Build history of the part. All positions in model axes, mm. A direction names the side the tool comes from. Round coordinates to 2 decimals unless told otherwise and drop trailing zeros. Write each loop counter-clockwise with the first axis right and the second up, starting at its lowest first coordinate (ties: lowest second). Pieces come first, ordered by that corner, then holes.
Item 1: Drop flat-ended pins along their axis: pin 1 Ø5.5 at (x, y) = (91, 2) entering from +Z; pin 2 Ø2.5 at (x, y) = (76, 6.5) entering from +Z; pin 3 Ø1.5 at (y, z) = (7.5, -17.5) entering from +X. Give the stop position or say it passes through.
Item 2: Band-saw the part on C-C, the plane x = -82. Write the cut outline in (y, z), then the cut area to 3 significant figures.
Item 3: Band-saw the part on B-B, the plane z = 73.5. Write the cut outline in (x, y), then the cut area to 4 significant figures.
Item 4: Wall check: probe 1 along Z at (x, y) = (82.6, 5.25); probe 2 along Y at (x, z) = (-52, 74.5); probe 3 along Z at (x, y) = (-14, 3.5). Give the ranges that are in metal, low to high.
Item 5: Mould opens along X. For faces 1 (the flat face through (71, 2, 70)), 2 (the flat face through (75, 7, 10.16)), 3 (the flat face through (11.425, 4.507, -23.224)) say: +X half, -X half, draft (parallel to the pull), parting line (faces both ways), or undercut.
Item 6: Band-saw the part on A-A, the plane x = 60. Write the cut outline in (y, z), then the cut area to 3 significant figures.
Item 7: Band-saw the part on D-D, the plane x = -29.5. Write the cut outline in (y, z), then the cut area to 3 significant figures.
Item 8: 3-axis set-ups, long thin cutter, end or side, ignore diameter. For faces 4 (the flat face through (-23.22, 4.51, -22.74)), 5 (the flat face through (75, 7, -23.851)), 6 (the flat face through (10.379, 2.028, -20.027)), 7 (the flat face through (75, 10, -7)), 8 (the flat face through (92, 3, 25.4)): which of +Z, -Z, +X, -X, +Y, -Y reach the whole face in a straight line?
Autodesk Inventor part; units mm, degrees
ref_plane "YZ Plane" through (0, 0, 0) normal (1, 0, 0) x (0, 1, 0)
ref_plane "XZ Plane" through (0, 0, 0) normal (0, 1, 0) x (-1, 0, 0)
ref_plane "XY Plane" through (0, 0, 0) normal (0, 0, 1) x (1, 0, 0)
sketch "Sketch1" plane through (0, 0, 0) normal (0, 1, 0) x (-1, 0, 0)
  line L0 (101.6, -101.6) -> (-101.6, -101.6)
  line L1 (-101.6, -101.6) -> (-101.6, 101.6)
  line L2 (-101.6, 101.6) -> (101.6, 101.6)
  line L3 (101.6, 101.6) -> (101.6, -101.6)
  line L4 (96.6, -96.6) -> (-96.6, -96.6)
  line L5 (-96.6, -96.6) -> (-96.6, 96.6)
  line L6 (-96.6, 96.6) -> (96.6, 96.6)
  line L7 (96.6, 96.6) -> (96.6, -96.6)
  line L8 (101.6, 101.6) -> (-40.4, 101.6)
  circle A0 centre (0, 0) radius 88.9
  line L9 (-40.4, 101.6) -> (-101.6, 40.4)
  line L10 (-45.4, 101.6) -> (-101.6, 45.4)
  line L11 (96.6, 96.6) -> (96.6, 101.6)
  line L12 (-45.4, 101.6) -> (-35.4, 101.6)
  line L13 (-35.4, 101.6) -> (-35.4, 96.6)
  line L14 (-35.4, 96.6) -> (-45.4, 96.6)
  line L15 (-45.4, 96.6) -> (-45.4, 101.6)
  line L16 (-101.6, 39.4) -> (-39.4, 101.6)
  line L17 (95.6, -95.6) -> (-95.6, -95.6)
  line L18 (-95.6, -95.6) -> (-95.6, 95.6)
  line L19 (-95.6, 95.6) -> (95.6, 95.6)
  line L20 (95.6, 95.6) -> (95.6, -95.6)
  point P0 (96.6, 51.2168)
  point P1 (101.6, 40.4)
  point P2 (101.6, -40.4)
  point P3 (96.6, -51.2168)
  point P4 (-96.6, 45.4)
  point P5 (-45.4, 96.6)
  point P6 (-45.4, 95.6)
  point P7 (-95.6, 45.4)
  dimension "d0" = 203.2
  dimension "d1" = 203.2
  dimension "d2" = 101.6
  dimension "d3" = 101.6
  dimension "d4" = 5
  dimension "d5" = 5
  dimension "d6" = 5
  dimension "d7" = 5
  dimension "d8" = 142
  dimension "d9" = 61.2
  dimension "d10" = 177.8
  dimension "d11" = 5
  dimension "d12" = 5
  dimension "d13" = 10
  dimension "d14" = 1
  dimension "d15" = 1
  dimension "d16" = 1
  dimension "d17" = 1
  dimension "d18" = 1
extrude "Extrusion1" add sketch "Sketch1" along normal blind 5 contours L16 L19 L20 L17 L18 | A0
sketch "Sketch2" plane through (0, 5, 0) normal (0, 1, 0) x (1, 0, 0)
  circle A0 centre (0, 0) radius 34.925
  circle A1 centre (0, 0) radius 88.9
  line L0 (0, 0) -> (53.5014, -70.9987)
  line L1 (0, 0) -> (70.9987, -53.5014)
  line L2 (45.4, -95.6) -> (95.6, -45.4)
  line L3 (70.5, -70.5) -> (0, 0)
  point P0 (21.0184, -27.8923)
  point P1 (27.8923, -21.0184)
  dimension "d21" = 69.85
  dimension "d22" = 177.8
  dimension "d23" = 8
  dimension "d24" = 8
extrude "Extrusion2" cut sketch "Sketch2" against normal blind 5 contours A0 L3 A1 L0 | L1 A1 L3 A0
sketch "Sketch3" plane through (0, 5, 0) normal (0, 1, 0) x (1, 0, 0)
  circle A0 centre (0, 0) radius 2.5
  line L0 (11.3314, 2.139) -> (-2.139, -11.3314)
  line L1 (0, 0) -> (-5.6569, 5.6569)
  line L2 (-5.6569, -14.8492) -> (-26.163, 5.6569)
  line L3 (-5.6569, 26.163) -> (14.8492, 5.6569)
  circle A1 centre (-5.6569, 5.6569) radius 14
  line L4 (-26.163, 5.6569) -> (-5.6569, 26.163)
  line L5 (14.8492, 5.6569) -> (-5.6569, -14.8492)
  line L6 (-40.3051, 5.6569) -> (-5.6569, 40.3051)
  line L7 (-5.6569, 40.3051) -> (28.9914, 5.6569)
  line L8 (28.9914, 5.6569) -> (-5.6569, -28.9914)
  line L9 (-5.6569, -28.9914) -> (-40.3051, 5.6569)
  line L10 (-22.6451, 9.1747) -> (-9.1747, 22.6451)
  line L11 (-9.1747, 22.6451) -> (-12.7668, 26.2372)
  line L12 (-12.7668, 26.2372) -> (-26.2372, 12.7668)
  line L13 (-26.2372, 12.7668) -> (-22.6451, 9.1747)
  line L14 (-36.0624, 5.6569) -> (-5.6569, 36.0624)
  line L15 (-5.6569, 36.0624) -> (26.8701, 3.5355)
  line L16 (26.8701, 3.5355) -> (-3.5355, -26.8701)
  line L17 (-3.5355, -26.8701) -> (-36.0624, 5.6569)
  arc A2 (-5.6569, -28.9914) -> (28.9914, 5.6569) centre (0.4206, -0.4206) ccw
  dimension "d27" = 8
  dimension "d28" = 28
  dimension "d29" = 29
  dimension "d30" = 29
  dimension "d31" = 14.5
  dimension "d32" = 10
  dimension "d33" = 10
  dimension "d34" = 10
  dimension "d35" = 10
  dimension "d36" = 5.08
  dimension "d37" = 9.525
  dimension "d38" = 9.525
  dimension "d39" = 3
  dimension "d40" = 3
  dimension "d41" = 0
  dimension "d42" = 3
  dimension "d51" = 29.21
extrude "Extrusion3" cut sketch "Sketch3" against normal blind 1 contours A0 | L0 L5 L2 L4 L3 | L4 L13 L12 L11 | A1 | L6 L7 L8 L15 L14 L17 L9 | L8 A2 | L17 L14 L15 L8
sketch "Sketch4" plane through (0, 4, 0) normal (0, 1, 0) x (1, 0, 0)
  line L0 (-36.0624, 5.6569) -> (-5.6569, 36.0624)
  line L1 (-5.6569, 36.0624) -> (26.8701, 3.5355)
  line L2 (26.8701, 3.5355) -> (-3.5355, -26.8701)
  line L3 (-3.5355, -26.8701) -> (-36.0624, 5.6569)
  line L4 (-5.6569, 40.3051) -> (28.9914, 5.6569)
  line L5 (-40.3051, 5.6569) -> (-5.6569, 40.3051)
  line L6 (-5.6569, -28.9914) -> (-40.3051, 5.6569)
  line L7 (28.9914, 5.6569) -> (-5.6569, -28.9914)
  arc A0 (-3.5355, -26.8701) -> (26.8701, 3.5355) centre (4.0877, -4.0877) ccw
  point P0 (0, 0)
  dimension "d45" = 3
  dimension "d46" = 3
  dimension "d47" = 3
  dimension "d48" = 0
extrude "Extrusion4" cut sketch "Sketch4" against normal blind 5 contours L0 L1 L2 L3 | L2 A0
sketch "Sketch6" plane through (0, 5, 0) normal (0, 1, 0) x (1, 0, 0)
  line L0 (95.6, 95.6) -> (-95.6, 95.6)
  line L1 (95.6, 95.6) -> (87.6, 95.6)
  line L2 (87.6, 95.6) -> (87.6, -46.4)
  line L3 (87.6, -46.4) -> (95.6, -46.4)
  line L4 (95.6, -46.4) -> (95.6, 95.6)
  line L5 (95.6, -45.4) -> (95.6, 95.6)
  line L6 (87.6, -25.4) -> (95.6, -25.4)
  line L7 (95.6, -25.4) -> (95.6, 50.8)
  line L8 (95.6, 50.8) -> (87.6, 50.8)
  line L9 (87.6, 50.8) -> (87.6, -25.4)
  line L10 (0, 0) -> (95.6, 0)
  dimension "d58" = 8
  dimension "d59" = 142
  dimension "d62" = 50.8
  dimension "d63" = 25.4
extrude "Extrusion6" cut sketch "Sketch6" against normal blind 25.4 contours L4 L10 L2 L8 | L4 L6 L2 L10
sketch "Sketch7" plane through (0, 5, 0) normal (0, 1, 0) x (1, 0, 0)
  line L0 (-95.6, 95.6) -> (-95.6, -95.6)
  line L1 (-95.6, -95.6) -> (45.4, -95.6)
  line L2 (95.6, 50.8) -> (87.6, 50.8)
  line L3 (87.6, 50.8) -> (62.2, 50.8)
  line L4 (87.6, -25.4) -> (87.6, 50.8)
  line L5 (87.6, -25.4) -> (87.6, 50.8)
  line L6 (87.6, 50.8) -> (95.6, 50.8)
  line L7 (87.6, 50.8) -> (62.2, 50.8)
  line L8 (62.2, 50.8) -> (62.2, -10.16)
  line L9 (62.2, -10.16) -> (87.6, -10.16)
  line L10 (87.6, -10.16) -> (87.6, 50.8)
  line L11 (62.2, 23.8506) -> (87.6, 23.8506)
  point P0 (0, 0)
  dimension "d72" = 60.96
  dimension "d90" = 34.0106
extrude "Extrusion7" add sketch "Sketch7" along normal blind 5 contours L4 L9 L8 L11
sketch "Sketch8" plane through (0, 10, 0) normal (0, 1, 0) x (1, 0, 0)
  line L0 (48.8597, -4.3723) -> (48.8597, 15.6277)
  line L1 (14.8597, -4.3723) -> (14.8597, 15.6277)
  line L2 (48.8597, 15.6277) -> (14.8597, 15.6277)
  line L3 (31.8597, 15.6277) -> (31.8597, -4.3723)
  circle A0 centre (31.8597, 10.6277) radius 1
  circle A1 centre (31.8597, 0.6277) radius 1
  line L4 (62.2, -10.16) -> (87.6, -10.16)
  line L5 (62.2, -10.16) -> (87.6, -10.16)
  line L6 (87.6, -10.16) -> (87.6, 6.8326)
  line L7 (87.6, 50.8) -> (87.6, -25.4)
  line L8 (87.6, 6.8326) -> (62.2, 6.8326)
  circle A2 centre (82.6, 6.8326) radius 1.5
  circle A3 centre (67.2, 6.8326) radius 1.5
  point P0 (0, 0)
  dimension "d73" = 2
  dimension "d74" = 2
  dimension "d75" = 5
  dimension "d76" = 5
  dimension "d77" = 17
  dimension "d78" = 16.9926
  dimension "d79" = 3
  dimension "d80" = 3
  dimension "d81" = 5
  dimension "d82" = 5
hole "Hole1" at (82.6, 10, -6.8326) at (67.2, 10, -6.8326) direction (0, -1, 0) diameter 2.85 depth 12.7 tip angle 118 countersink diameter 3.175 countersink angle 82
equation "\"d1\" = d0"
properties part number "Drop_Plate"
Results:
1. pin 1: stops at z = 52.75
1. pin 2: stops at z = 10.16
1. pin 3: stops at x = 87.6
2. outline: (0, -95.6) - (5, -95.6) - (5, 95.6) - (0, 95.6) - close
2. area: 956 mm2
3. outline: (-95.6, 0) - (67.5, 0) - (67.5, 5) - (-95.6, 5) - close
3. area: 815.5 mm2
4. probe 1: z = -23.85 to -8.26, -5.41 to 10.16
4. probe 2: y = 0 to 5
4. probe 3: z = -95.6 to -27.72, 16.41 to 95.6
5. face 1: +X half
5. face 2: draft
5. face 3: undercut
6. outline: (0, -95.6) - (5, -95.6) - (5, 45.21) - (0, 45.21) - close; (0, 65.6) - (5, 65.6) - (5, 81) - (0, 81) - close
6. area: 781 mm2
7. outline: (0, -95.6) - (5, -95.6) - (5, -16.46) - (4, -16.46) - (4, -12.22) - (0, -12.22) - close; (0, 0.91) - (4, 0.91) - (4, 5.15) - (5, 5.15) - (5, 95.6) - (0, 95.6) - close
7. area: 882 mm2
8. face 4: +Y
8. face 5: -Z, +X, -X, +Y
8. face 6: +Y, -Y
8. face 7: +Z, -Z, +X, -X, +Y
8. face 8: +X, +Y, -Y
